from build123d import *

# Parameters (mm, degrees)
SKETCH_1_R             = 11
EXTRUDE_1_DEPTH        = 3.475
SKETCH_3_R             = 10
SKETCH_3_R_2           = 9.75
CUT_EXTRUDE_2_DEPTH    = 0.5
FILLET_4_R             = 0.5
SKETCH_7_R             = 4
CUT_EXTRUDE_3_DEPTH    = 16.939749841
SKETCH_15_R            = 5
EXTRUDE_7_DEPTH        = 0.1
SKETCH_18_R            = 4
CUT_EXTRUDE_4_DEPTH    = 16.961849047
FILLET_4_OF_MIRROR_3_R = 0.5
SKETCH_19_R            = 4
CUT_EXTRUDE_5_DEPTH    = 18.120820658


with BuildPart() as part:
    # Эскиз1 → Бобышка-Вытянуть1 (new body)
    with BuildSketch(Plane(origin=(0, 0, 0), x_dir=(1, 0, 0), z_dir=(0, 1, 0))):
        with Locations(Location((0, 0, 0), (0, 0, 270))):
            Circle(SKETCH_1_R)
    extrude_1 = extrude(amount=EXTRUDE_1_DEPTH)

    # Эскиз3 → Вырез-Вытянуть2 (cut)
    with BuildSketch(Plane.XZ):
        with Locations(Location((0, 0, 0), (0, 0, 270))):
            Circle(SKETCH_3_R)
        with Locations(Location((0, 0, 0), (0, 0, 270))):
            Circle(SKETCH_3_R_2, mode=Mode.SUBTRACT)
    cut_extrude_2 = extrude(amount=-CUT_EXTRUDE_2_DEPTH, mode=Mode.SUBTRACT)

    # Скругление4
    # the kernel refuses this fillet: 0.5 mm, written as the material it adds along each edge
    with BuildSketch(Plane(origin=(0, 0.5, 0), x_dir=(0, 0, -1), z_dir=(-1, 0, 0))) as fillet_4_piece_1:
        with BuildLine():
            CenterArc((9.5, 0.433012702), FILLET_4_R, 300, 60)
            Line((9.75, 0), (9.755, -0.008660254))
            ThreePointArc((9.755, -0.008660254), (9.875, -0.01), (10, -0.01))
            Line((10, -0.01), (10.01, 0))
            Line((10.01, 0), (10.01, 0.433012702))
            Line((10.01, 0.433012702), (10, 0.433012702))
        make_face()
    revolve(axis=Axis((0, 0.5, 0), (0, -1, 0)))

    # Фаска1: read off the stored shape, not the designer's step
    # Фаска1 outline → Фаска1 (revolve, cut)
    with BuildSketch(Plane.XY):
        with BuildLine():
            Line((9.25, 0.5), (8.75, 0))
            Line((8.75, 0), (9.75, 0))
            Line((9.75, 0), (9.75, 0.5))
            ThreePointArc((9.75, 0.5), (9.5, 0.566987298), (9.25, 0.5))
        make_face()
    chamfer_1 = revolve(axis=Axis((0, 0, 0), (0, 1, 0)), mode=Mode.SUBTRACT)

    # Эскиз7 → Вырез-Вытянуть3 (cut, symmetric)
    with BuildSketch(Plane.XZ):
        with Locations(Location((0, 0, 0), (0, 0, 270))):
            Circle(SKETCH_7_R)
    cut_extrude_3 = extrude(amount=CUT_EXTRUDE_3_DEPTH, both=True, mode=Mode.SUBTRACT)

    # Эскиз15 → Бобышка-Вытянуть7 (add)
    with BuildSketch(Plane.XZ):
        with Locations(Location((0, 0, 0), (0, 0, 90))):
            Circle(SKETCH_15_R)
    extrude_7 = extrude(amount=EXTRUDE_7_DEPTH)

    # Эскиз18 → Вырез-Вытянуть4 (cut, through all)
    with BuildSketch(Plane.XZ.offset(0.1)):
        with Locations(Location((0, 0, 0), (0, 0, 270))):
            Circle(SKETCH_18_R)
    extrude(amount=-CUT_EXTRUDE_4_DEPTH, mode=Mode.SUBTRACT)

    # Зеркальное отражение3: Бобышка-Вытянуть1, Вырез-Вытянуть2, Фаска1, Вырез-Вытянуть3, Бобышка-Вытянуть7 across plane
    add(extrude_1.mirror(Plane.ZX.offset(3.475)))
    add(cut_extrude_2.mirror(Plane.ZX.offset(3.475)), mode=Mode.SUBTRACT)
    add(chamfer_1.mirror(Plane.ZX.offset(3.475)), mode=Mode.SUBTRACT)
    add(cut_extrude_3.mirror(Plane.ZX.offset(3.475)), mode=Mode.SUBTRACT)
    add(extrude_7.mirror(Plane.ZX.offset(3.475)))

    # Скругление4 of Зеркальное отражение3
    # the kernel refuses this fillet: 0.5 mm, written as the material it adds along each edge
    with BuildSketch(Plane(origin=(0, 6.45, 0), x_dir=(0, 0, -1), z_dir=(-1, 0, 0))) as fillet_4_of_mirror_3_piece_1:
        with BuildLine():
            CenterArc((9.5, -0.433012702), FILLET_4_OF_MIRROR_3_R, 0, 60)
            Line((9.75, 0), (9.755, 0.008660254))
            ThreePointArc((9.755, 0.008660254), (9.875, 0.01), (10, 0.01))
            Line((10, 0.01), (10.01, 0))
            Line((10.01, 0), (10.01, -0.433012702))
            Line((10.01, -0.433012702), (10, -0.433012702))
        make_face()
    revolve(axis=Axis((0, 6.45, 0), (0, -1, 0)))

    # Эскиз19 → Вырез-Вытянуть5 (cut, through all)
    with BuildSketch(Plane(origin=(0, 7.05, 0), x_dir=(1, 0, 0), z_dir=(0, 1, 0))):
        with Locations(Location((0, 0, 0), (0, 0, 90))):
            Circle(SKETCH_19_R)
    extrude(amount=-CUT_EXTRUDE_5_DEPTH, mode=Mode.SUBTRACT)


solid = part.part
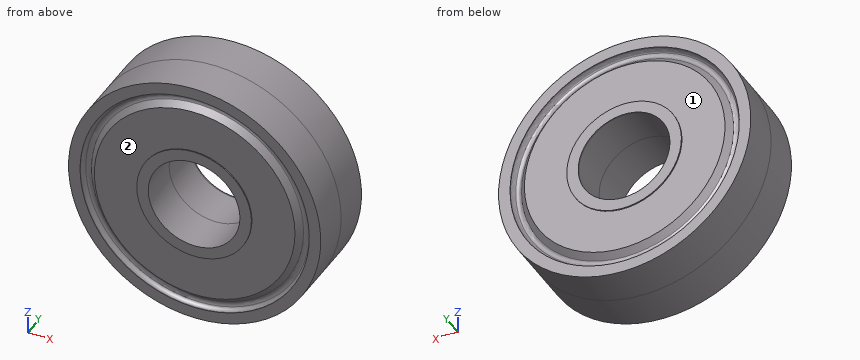
Build history of the part. All positions in model axes, mm. Face numbers are marked on the shaded views. A direction names the side the tool comes from. Give positions to 0.01 mm unless a question says otherwise; leave off trailing zeros. Loops run counter-clockwise (first coordinate to the right, second up) from the corner with the lowest first, then second, coordinate; pieces in that order, holes last. Notation, with made-up numbers: (43, 85.5) -> (89, 85.5) arc R9 cw to (89, 95.5) -> close; hole circle Ø4 at (83, 66.5). An arc over 180 degrees is marked (long way). Answer in a Markdown table with one row per item.
Item 1: Probe line 1 along X through (y, z) = (5.15, 0); line 2 along X through (y, z) = (7, 0); line 3 along Y through (x, z) = (-1, 10). List the from-to ranges inside material, lowest first. Write a range as [from, to].
Findings below:
| item | result |
|---|---|
| line 1 | x = [-11, -4], [4, 11] |
| line 2 | x = [-5, -4], [4, 5] |
| line 3 | y = [0, 6.95] |
Item 2: Flat gauge pins, fed straight in: P1, Ø5, axis at x = -8.5, z = 1.5, coming from the -Y side; P2, Ø2, axis at y = 1.5, z = 4, coming from the +X side; P3, Ø4, axis at x = -4, y = 5, coming from the +Z side. Where does each tip first touch, or does it go through?
Findings below:
| item | result |
|---|---|
| P1 | stops at y = 0 |
| P2 | stops at x = 10.58 |
| P3 | stops at z = 10.82 |
Item 3: Slice it at A-A on y = 4.25. Write the cut outline in (x, z).
Findings below:
| item | result |
|---|---|
| outline | circle Ø22 at (0, 0); hole circle Ø8 at (0, 0) |
Item 4: Tool access for the marked faces 1 and 2: list every direction of +Z, -Z, +X, -X, +Y, -Y with a clear straight run to the whole face (end or side of a thin tool).
Findings below:
| item | result |
|---|---|
| face 1 | +Y |
| face 2 | -Y |
